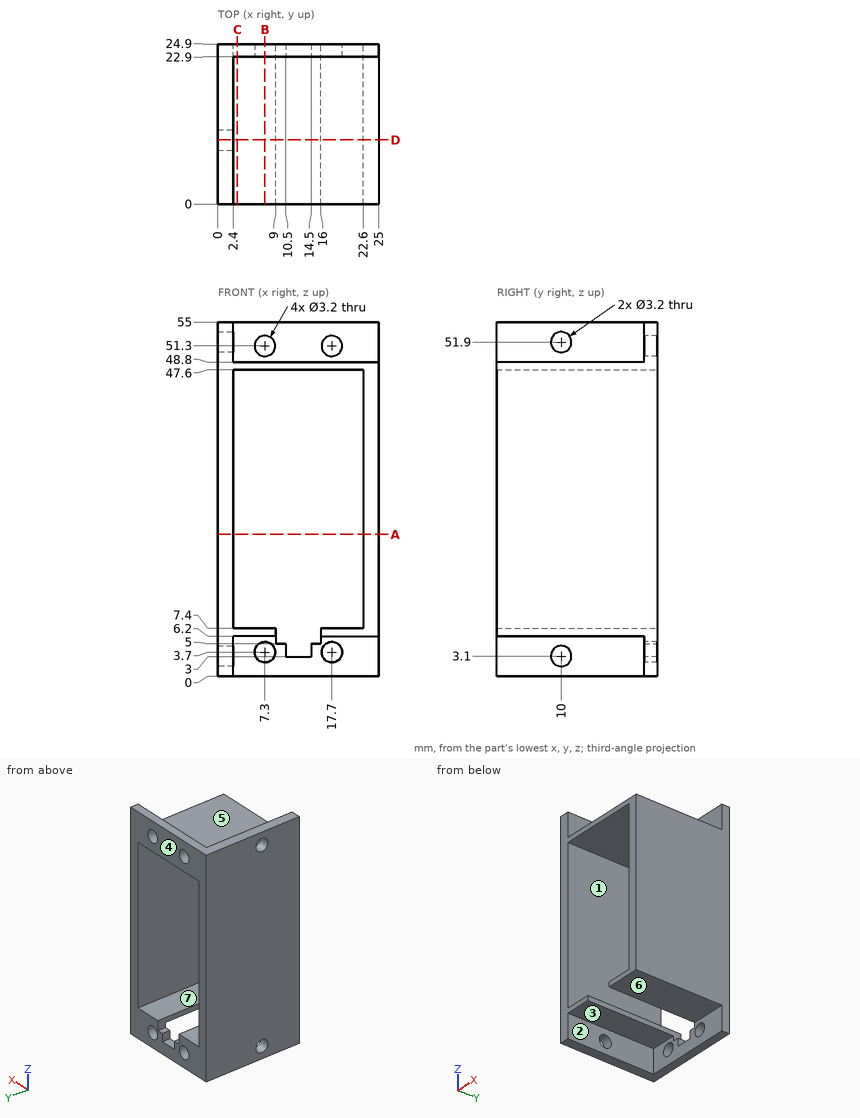
Input: dimensioned drawing with shaded views. Units: mm. Origin: part minimum x, y, z. A direction names the side the tool comes from. Round coordinates to 2 decimals unless told otherwise and drop trailing zeros. Order: outer loops, then holes, each group sorted by start corner. A loop starts at its lowest first (then second) coordinate and runs counter-clockwise, first axis right, second up.
1. Cut plane A-A, the plane z = 22. Output: boundary loops of the cut face in (x, y).
The answers:
outline: (0, 0) - (2.4, 0) - (2.4, 24.9) - (0, 24.9) - close; (22.6, 0) - (25, 0) - (25, 24.9) - (22.6, 24.9) - close
2. Cut plane D-D, the plane y = 10. Output: boundary loops of the cut face in (x, z), then the cut area to 3 significant figures.
The answers:
outline: (0, 0) - (2.4, 0) - (2.4, 1.5) - (0, 1.5) - close; (0, 4.7) - (2.4, 4.7) - (2.4, 6.2) - (9, 6.2) - (9, 7.4) - (2.4, 7.4) - (2.4, 47.6) - (22.6, 47.6) - (22.6, 7.4) - (16, 7.4) - (16, 6.2) - (25, 6.2) - (25, 48.8) - (2.4, 48.8) - (2.4, 50.3) - (0, 50.3) - close; (0, 53.5) - (2.4, 53.5) - (2.4, 55) - (0, 55) - close
area: 259 mm2
3. Material intervals for line 1 (Z direction, x = 7.3, y = 23.65); line 2 (Z direction, x = 8, y = 17); line 3 (X direction, y = 2.5, z = 19), sorted ascending.
The answers:
line 1: z = 0 to 2.1, 5.3 to 7.4, 47.6 to 49.7, 52.9 to 55
line 2: z = 6.2 to 7.4, 47.6 to 48.8
line 3: x = 0 to 2.4, 22.6 to 25
4. Mould query, pull axis Z, two halves, no side actions, for the marked faces 1, 2 and 3. Classes: released by +Z, released by -Z, zero draft, split by the parting line, or undercut.
The answers:
face 1: undercut
face 2: zero draft
face 3: released by -Z
5. Cut plane B-B, the plane x = 7.3. Output: boundary loops of the cut face in (y, z), then the cut area to 3 significant figures.
The answers:
outline: (0, 6.2) - (22.9, 6.2) - (22.9, 5.3) - (24.9, 5.3) - (24.9, 7.4) - (0, 7.4) - close; (0, 47.6) - (24.9, 47.6) - (24.9, 49.7) - (22.9, 49.7) - (22.9, 48.8) - (0, 48.8) - close; (22.9, 0) - (24.9, 0) - (24.9, 2.1) - (22.9, 2.1) - close; (22.9, 52.9) - (24.9, 52.9) - (24.9, 55) - (22.9, 55) - close
area: 71.8 mm2
6. Set-up query: the marked faces 4, 5, 6 and 7. Return all of +Z, -Z, +X, -X, +Y, -Y with unobstructed straight access to the full face (end or side cutting, diameter ignored); none if empty.
The answers:
face 4: +Z, -Z, +X, -X, +Y
face 5: +Z, +X, -Y
face 6: -Z, +X, -Y
face 7: +Y, -Y
7. Cut plane C-C, the plane x = 3. Output: boundary loops of the cut face in (y, z), then the cut area to 3 significant figures.
The answers:
outline: (0, 6.2) - (22.9, 6.2) - (22.9, 0) - (24.9, 0) - (24.9, 7.4) - (0, 7.4) - close; (0, 47.6) - (24.9, 47.6) - (24.9, 55) - (22.9, 55) - (22.9, 48.8) - (0, 48.8) - close
area: 84.6 mm2
8. Pin query (flat end, axial travel): P1, Ø4, axis at x = 6.5, y = 19, coming from the +Z side; P2, Ø1.9, axis at y = 13.5, z = 50.5, coming from the +X side; P3, Ø7, axis at x = 22, y = 5.5, coming from the -Z side. Return the tip coordinate at first contact, or that it passes through.
The answers:
P1: stops at z = 48.8
P2: stops at x = 2.4
P3: stops at z = 6.2
